```python
from build123d import *

# Parameters (mm, degrees)
SKETCH1_W           = 60
SKETCH1_H           = 60
SKETCH1_R           = 17.75
SKETCH1_W_2         = 10
SKETCH1_H_2         = 6
SKETCH1_W_3         = 6
SKETCH1_H_3         = 10
BOSS_EXTRUDE1_DEPTH = 6


with BuildPart() as part:
    # Sketch1 → Boss-Extrude1 (new body)
    # profile 1 of 9: a face of its own
    with BuildSketch(Plane(origin=(0, 0, 0), x_dir=(1, 0, 0), z_dir=(0, 1, 0))):
        Rectangle(SKETCH1_W, SKETCH1_H)
        with Locations(Location((0, 0, 0), (0, 0, 270))):
            Circle(SKETCH1_R, mode=Mode.SUBTRACT)
    # profile 2 of 9: a face of its own
    with BuildSketch(Plane(origin=(0, 0, 0), x_dir=(1, 0, 0), z_dir=(0, 1, 0))):
        with Locations((15, -33)):
            Rectangle(SKETCH1_W_2, SKETCH1_H_2)
    # profile 3 of 9: a face of its own
    with BuildSketch(Plane(origin=(0, 0, 0), x_dir=(1, 0, 0), z_dir=(0, 1, 0))):
        with Locations((-15, -33)):
            Rectangle(SKETCH1_W_2, SKETCH1_H_2)
    # profile 4 of 9: a face of its own
    with BuildSketch(Plane(origin=(0, 0, 0), x_dir=(1, 0, 0), z_dir=(0, 1, 0))):
        with Locations((-33, -15)):
            Rectangle(SKETCH1_W_3, SKETCH1_H_3)
    # profile 5 of 9: a face of its own
    with BuildSketch(Plane(origin=(0, 0, 0), x_dir=(1, 0, 0), z_dir=(0, 1, 0))):
        with Locations((-33, 15)):
            Rectangle(SKETCH1_W_3, SKETCH1_H_3)
    # profile 6 of 9: a face of its own
    with BuildSketch(Plane(origin=(0, 0, 0), x_dir=(1, 0, 0), z_dir=(0, 1, 0))):
        with Locations((-15, 33)):
            Rectangle(SKETCH1_W_2, SKETCH1_H_2)
    # profile 7 of 9: a face of its own
    with BuildSketch(Plane(origin=(0, 0, 0), x_dir=(1, 0, 0), z_dir=(0, 1, 0))):
        with Locations((15, 33)):
            Rectangle(SKETCH1_W_2, SKETCH1_H_2)
    # profile 8 of 9: a face of its own
    with BuildSketch(Plane(origin=(0, 0, 0), x_dir=(1, 0, 0), z_dir=(0, 1, 0))):
        with Locations((33, 15)):
            Rectangle(SKETCH1_W_3, SKETCH1_H_3)
    # profile 9 of 9: a face of its own
    with BuildSketch(Plane(origin=(0, 0, 0), x_dir=(1, 0, 0), z_dir=(0, 1, 0))):
        with Locations((33, -15)):
            Rectangle(SKETCH1_W_3, SKETCH1_H_3)
    extrude(amount=BOSS_EXTRUDE1_DEPTH)


solid = part.part
```
Geometry: final body of the model. Coordinates: model frame, mm. A direction names the side the tool comes from. Give positions to 0.01 mm unless a question says otherwise; leave off trailing zeros. Loops run counter-clockwise (first coordinate to the right, second up) from the corner with the lowest first, then second, coordinate; pieces in that order, holes last. Notation, with made-up numbers: (40, 50.5) -> (65, 50.5) arc R18 cw to (65, 68.5) -> close; hole circle Ø10 at (55, 24). An arc over 180 degrees is marked (long way). Use one line per item in the form item = value.
Item 1: Section query A-A on z = 0. Output: boundary loops of the cut face in (x, y), and give its area (3 significant figures).
A:
outline = (-30, 0) -> (-17.75, 0) -> (-17.75, 6) -> (-30, 6) -> close; (17.75, 0) -> (30, 0) -> (30, 6) -> (17.75, 6) -> close
area = 147 mm^2
Item 2: Draft query along X for faces 5 (the face through (33, 3, -20)), 6 (the face through (0, 3, -30)), 7 (the face through (20, 3, -33)). Return one class per face: pulls with the +X half, pulls with the -X half, needs draft (parallel to the pull), parting line crosses it, or undercut.
A:
face_5 = needs draft
face_6 = undercut
face_7 = pulls with the +X half
Item 3: Section query C-C on z = 22.5. Output: boundary loops of the cut face in (x, y), and give its area (3 significant figures).
A:
outline = (-30, 0) -> (30, 0) -> (30, 6) -> (-30, 6) -> close
area = 360 mm^2
Item 4: Section query B-B on x = 0. Output: boundary loops of the cut face in (y, z), and give its area (3 significant figures).
A:
outline = (0, -30) -> (6, -30) -> (6, -17.75) -> (0, -17.75) -> close; (0, 17.75) -> (6, 17.75) -> (6, 30) -> (0, 30) -> close
area = 147 mm^2
Item 5: Section query D-D on x = -26. Output: boundary loops of the cut face in (y, z).
A:
outline = (0, -30) -> (6, -30) -> (6, 30) -> (0, 30) -> close
Item 6: Pin query (flat end, axial travel): P1, Ø1.8, axis at y = 4, z = 26, coming from the -X side; P2, Ø1.8, axis at x = 33.5, y = 1.5, coming from the +Z side; P3, Ø3, axis at y = 3.5, z = -32, coming from the +X side. Return the tip coordinate at first contact, or that it passes through.
A:
P1 = -30
P2 = 20
P3 = 20
Item 7: Line query: probe 1 along X at (y, z) = (4.7, -32); probe 2 along X at (y, z) = (4.7, 0); probe 3 along Z at (x, y) = (-28.5, 5.15). Output: solid intervals per line, ascending.
A:
probe_1 = -20 to -10, 10 to 20
probe_2 = -30 to -17.75, 17.75 to 30
probe_3 = -30 to 30
Item 8: Access query for faces 1 (the face through (-33, 3, -20)), 2 (the face through (30, 3, 25)), 3 (the face through (33, 3, -10)), 4 (the face through (25, 3, -30)). Directions: +Z, -Z, +X, -X, +Y, -Y. A direction counts if a zero-diameter tool reaches every point of the face in a straight line with its end or side. Return the directions, or none.
A:
face_1 = -Z, -X, +Y, -Y
face_2 = +Z, +X, +Y, -Y
face_3 = +X, +Y, -Y
face_4 = -Z, +X, +Y, -Y
